from build123d import *

# Parameters (mm, degrees)
F0_R      = 22.5
F1_DEPTH  = 35
F2_R      = 18
F3_DEPTH  = 8
F5_D      = 25
F5_DEPTH  = 20
F5_TIP    = 7.5107577378
F6_D      = 20
F8_D      = 2.2
F8_DEPTH  = 15
F8_TIP    = 0.6609466809
F9_W      = 60.0066725165
F9_H      = 50.9474342689
F10_DEPTH = 25


with BuildPart() as f1:
    # F0 (on Top) → F1 (new body)
    with BuildSketch(Plane.XY):
        Circle(F0_R)
    extrude(amount=F1_DEPTH)

    # F2 (on face) → F3 (cut)
    with BuildSketch(Plane(origin=(0, 0, 0), x_dir=(1, 0, 0), z_dir=(0, 0, -1))):
        Circle(F2_R)
    extrude(amount=-F3_DEPTH, mode=Mode.SUBTRACT)

    # F5
    with Locations(Plane.XY.offset(35)):
        with Locations((0, 0)):
            Hole(F5_D / 2, depth=F5_DEPTH)
            with Locations((0, 0, -(F5_DEPTH + F5_TIP / 2))):  # 118° drill point
                Cone(0, F5_D / 2, F5_TIP, mode=Mode.SUBTRACT)

    # F6 (through all)
    with Locations(Plane.XY.offset(35)):
        with Locations((0, 0)):
            Hole(F6_D / 2)

    # F8
    with Locations(Plane.XY.offset(35)):
        with Locations((20, 0), (-10, 17.3205080757), (-10, -17.3205080757)):
            Hole(F8_D / 2, depth=F8_DEPTH)
            with Locations((0, 0, -(F8_DEPTH + F8_TIP / 2))):  # 118° drill point
                Cone(0, F8_D / 2, F8_TIP, mode=Mode.SUBTRACT)

    # F9 (on Front) → F10 (cut)
    with BuildSketch(Plane.XZ):
        with Locations((-0.6993999705, 19.8549819179)):
            Rectangle(F9_W, F9_H)
    extrude(amount=-F10_DEPTH, mode=Mode.SUBTRACT)


solid = f1.part
CAD build for the part. Positions are in the model's coordinates, mm. A direction names the side the tool comes from. Give positions to 0.01 mm unless a question says otherwise; leave off trailing zeros. Loops run counter-clockwise (first coordinate to the right, second up) from the corner with the lowest first, then second, coordinate; pieces in that order, holes last. Notation, with made-up numbers: M -2.5,47.5 L 54.5,47.5 A21 cw 54.5,53.5 Z; hole C -15,48.25 d11. An arc over 180 degrees is marked long. Answer in a Markdown table with one row per item. Add a question column.
Item 1: Band-saw the part on A-A on x = 0. Give the cut face in (y, z).
Item 2: Band-saw the part on C-C on z = 7. Give the cut face in (x, y), then the cut area to 3 significant figures.
Item 3: Probe probe 1 along Z at (x, y) = (13, -11.75); probe 2 along X at (y, z) = (-3.5, 8.5); probe 3 along X at (y, z) = (-3.25, 4.5). List the from-to ranges inside material, lowest first.
Item 4: Band-saw the part on B-B on z = 24.5. Give the cut face in (x, y).
Item 5: Tool access for faces 4 (the face through (20, -1.1, 27.4)), 5 (the face through (-18, 0, 18)), 6 (the face through (-10.5, -18.3, 27.4)), 7 (the face through (0, -10, 11)), 8 (the face through (0, -18, 4)): list every direction of +Z, -Z, +X, -X, +Y, -Y with a clear straight run to the whole face (end or side of a thin tool).
Item 6: Mould opens along X. For faces 1 (the face through (-0.22, -10.15, 13.59)), 2 (the face through (0, -14, 35)), 3 (the face through (-0.495, -22.495, 17.255)) say: +X half, -X half, draft (parallel to the pull), parting line (faces both ways), or undercut.
Item 7: Drop flat-ended pins along their axis: P1, Ø3, axis at x = 8, z = 30.5, coming from the -Y side; P2, Ø8, axis at y = -7.5, z = 11, coming from the +X side; P3, Ø3, axis at y = -15.5, z = 22, coming from the -X side. Give the stop position or say it passes through.
Item 8: Band-saw the part on D-D on x = 20. Give the cut face in (y, z), then the cut area to 3 significant figures.
Reply:
| question | item | result |
|---|---|---|
| 1 | outline | M -22.5,0 L -18,0 L -18,8 L -10,8 L -10,13.5 L -12.5,15 L -12.5,35 L -22.5,35 Z |
| 2 | outline | M -22.5,0 A22.5 ccw 22.5,0 L 18,0 A18 cw -18,0 Z |
| 2 | area | 286 mm^2 |
| 3 | probe 1 | z = 8 to 35 |
| 3 | probe 2 | x = -22.23 to -9.37, 9.37 to 22.23 |
| 3 | probe 3 | x = -22.26 to -17.7, 17.7 to 22.26 |
| 4 | outline | M -22.5,0 A22.5 ccw 22.5,0 L 21.1,0 A1.1 cw 18.9,0 L 12.5,0 A12.5 cw -12.5,0 Z; hole C -10,-17.32 d2.2 |
| 5 | face 4 | +Z, +Y |
| 5 | face 5 | +Z, -Z, +X, -X, +Y |
| 5 | face 6 | +Z |
| 5 | face 7 | +Z, -Z, +Y |
| 5 | face 8 | -Z, +Y |
| 6 | face 1 | undercut |
| 6 | face 2 | draft |
| 6 | face 3 | parting line |
| 7 | P1 | stops at y = -21.54 |
| 7 | P2 | stops at x = 22.23 |
| 7 | P3 | stops at x = -17.61 |
| 8 | outline | M -10.31,0 L 0,0 L 0,19.34 L -1.1,20 L -1.1,35 L -10.31,35 Z |
| 8 | area | 344 mm^2 |
